CAD build for the part. Positions are in the model's coordinates, mm. A direction names the side the tool comes from. Round coordinates to 2 decimals unless told otherwise and drop trailing zeros. Order: outer loops, then holes, each group sorted by start corner. A loop starts at its lowest first (then second) coordinate and runs counter-clockwise, first axis right, second up. Notation, with made-up numbers: M 56,66 L 73,66 A30 cw 73,97 Z; hole C -35,87.5 d6. An arc over 180 degrees is marked long. Put each result on its own line as item: value.
```python
from build123d import *

# Parameters (mm, degrees)
F1_DEPTH = 140
F2_T     = -2
F4_DEPTH = 4


with BuildPart() as f1:
    # F0 (on Top) → F1 (new body)
    with BuildSketch(Plane.XY):
        Polygon((0, -15.047), (13.031084, -7.5235), (13.031084, 7.5235), (0, 15.047), (-13.031084, 7.5235), (-13.031084, -7.5235), align=None)
    extrude(amount=F1_DEPTH)

    # F2
    f2_openings = [f1.faces().sort_by_distance(p)[0] for p in [
        (0, 0, 0),
    ]]
    offset(amount=F2_T, openings=f2_openings)

    # F3 (on face) → F4 (join)
    with BuildSketch(Plane.XY.offset(140)):
        Polygon((0, -11.047), (9.566983, -5.5235), (9.566983, 5.5235), (0, 11.047), (-9.566983, 5.5235), (-9.566983, -5.5235), align=None)
    extrude(amount=F4_DEPTH)


solid = f1.part
```
Item 1: Band-saw the part on B-B on x = -5. Give the cut face in (y, z).
Answers below:
outline: M -12.16,0 L -9.85,0 L -9.85,138 L 9.85,138 L 9.85,0 L 12.16,0 L 12.16,140 L 8.16,140 L 8.16,144 L -8.16,144 L -8.16,140 L -12.16,140 Z
Item 2: Tool access for faces 5 (the flat face through (-9.567, 0, 142)), 6 (the flat face through (0, 0, 144)), 7 (the flat face through (-4.85, -8.247, 141.972)), 8 (the flat face through (-5.438, 9.598, 68.034)), 9 (the flat face through (-4, -9, 140)): list every direction of +Z, -Z, +X, -X, +Y, -Y with a clear straight run to the whole face (end or side of a thin tool).
Answers below:
face 5: +Z, -X, +Y, -Y
face 6: +Z, +X, -X, +Y, -Y
face 7: +Z, -X, -Y
face 8: -Z
face 9: +Z
Item 3: Band-saw the part on A-A on z = 11. Give the cut face in (x, y).
Answers below:
outline: M -13.03,-7.52 L 0,-15.05 L 13.03,-7.52 L 13.03,7.52 L 0,15.05 L -13.03,7.52 Z; hole M -11.03,-6.37 L 0,-12.74 L 11.03,-6.37 L 11.03,6.37 L 0,12.74 L -11.03,6.37 Z
Item 4: Pin check, flat tips, straight feed: P1, Ø1, axis at x = -10, y = -5.5, coming from the -Z side; P2, Ø5, axis at x = 3.5, z = 42, coming from the -Y side; P3, Ø3, axis at y = 2, z = 142.5, coming from the -X side. Stop position of each tip, or through.
Answers below:
P1: z = 138
P2: y = -14.47
P3: x = -9.57
Item 5: Band-saw the part on C-C on y = 4. Give the cut face in (x, z), and give its area (3 significant figures).
Answers below:
outline: M -13.03,0 L -11.03,0 L -11.03,138 L 11.03,138 L 11.03,0 L 13.03,0 L 13.03,140 L 9.57,140 L 9.57,144 L -9.57,144 L -9.57,140 L -13.03,140 Z
area: 681 mm²
Item 6: Mould opens along Y. For faces 1 (the flat face through (5.438, -9.598, 68.034)), 2 (the flat face through (6.42, -11.34, 69.02)), 3 (the flat face through (4.85, 8.247, 141.972)), 4 (the flat face through (9.567, 0, 142)) say: pulls with the +Y half, pulls with the -Y half, needs draft (parallel to the pull), parting line crosses it, or undercut.
Answers below:
face 1: undercut
face 2: pulls with the -Y half
face 3: pulls with the +Y half
face 4: needs draft
Item 7: Probe line 1 along X through (y, z) = (3, 22); line 2 along Z through (x, y) = (2.75, 4); line 3 along Z through (x, y) = (-4, 11). List the from-to ranges inside material, lowest first. Write a range as [from, to].
Answers below:
line 1: [-13.03, -11.03], [11.03, 13.03]
line 2: [138, 144]
line 3: [0, 140]
